Part model, mm, in its own coordinate system. Face numbers are marked on the shaded views. A direction names the side the tool comes from. Round coordinates to 2 decimals unless told otherwise and drop trailing zeros. Write each loop counter-clockwise with the first axis right and the second up, starting at its lowest first coordinate (ties: lowest second). Pieces come first, ordered by that corner, then holes.
from build123d import *

# Parameters (mm, degrees)
SKETCH1_R           = 6.25
BOSS_EXTRUDE1_DEPTH = 3.75
BOSS_EXTRUDE2_DEPTH = 2.5


with BuildPart() as part:
    # Sketch1 → Boss-Extrude1 (new body, symmetric)
    with BuildSketch(Plane.XY):
        with BuildLine():
            ThreePointArc((14.68337521, -5), (23.5795956, -2.206380053), (19, 5.916079783))
            Line((19, 5.916079783), (1.5, 8.874119675))
            ThreePointArc((1.5, 8.874119675), (-1.711171484, 8.835830021), (-4.704473056, 7.672544119))
            ThreePointArc((-4.704473056, 7.672544119), (-14.388421791, 5.006214545), (-23.453994607, 0.681452586))
            Line((-23.453994607, 0.681452586), (-24.470827362, 2.403675322))
            Line((-24.470827362, 2.403675322), (-34.804163773, -3.697321205))
            Line((-34.804163773, -3.697321205), (-29.72, -12.308434881))
            ThreePointArc((-29.72, -12.308434881), (-19.025686771, -7.501050673), (-7.617535769, -4.793031276))
            ThreePointArc((-7.617535769, -4.793031276), (-1.570247279, -8.861959348), (5.50692712, -7.118549971))
            Line((5.50692712, -7.118549971), (14.68337521, -5))
        make_face()
        Circle(SKETCH1_R, mode=Mode.SUBTRACT)
    extrude(amount=BOSS_EXTRUDE1_DEPTH, both=True)

    # Sketch2 → Boss-Extrude2 (add, symmetric)
    with BuildSketch(Plane.XY):
        with BuildLine():
            Line((-28.63346637, -11.690418156), (-24.131806399, -9.129888895))
            Line((-24.131806399, -9.129888895), (-23.968684666, -9.421327611))
            Line((-23.968684666, -9.421327611), (-21.496617767, -13.767462129))
            ThreePointArc((-21.496617767, -13.767462129), (-22.466751825, -17.296987603), (-25.996277299, -16.326853546))
            Line((-25.996277299, -16.326853546), (-28.63346637, -11.690418156))
        make_face()
    extrude(amount=BOSS_EXTRUDE2_DEPTH, both=True)


solid = part.part
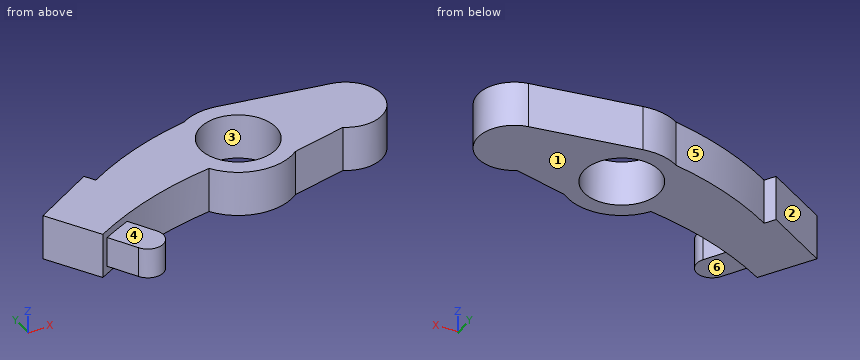
Q1. Saw through at A-A, the plane z = 1. Write the cut outline in (x, y).
Q2. Two-plate mould, pull along X, no slides. Class the marked faces 1, 2 and 3: released by +X, released by -X, zero draft, split by the parting line, or undercut.
Q3. Saw through at D-D, the plane x = 12.5. Write the cut outline in (y, z).
Q4. Saw through at C-C, the plane y = 3.75. Write the cut outline in (x, z), and give its area (3 significant figures).
Q5. Wall check: line 1 (Y direction, x = 0, z = -1.75); line 2 (X direction, y = -3, z = 1.25); line 3 (Y direction, x = -4, z = -0.5). Give the ranges that are in metal, low to high.
Q6. Drop flat-ended pins along their axis: P1, Ø1.5, axis at y = -8, z = 1.5, coming from the -X side; P2, Ø2, axis at x = -15, z = 0.5, coming from the +Y side; P3, Ø6, axis at x = -24, y = -15.5, coming from the +Z side. Give the stop position or say it passes through.
Q7. Tool access for the marked faces 4, 5 and 6: list every direction of +Z, -Z, +X, -X, +Y, -Y with a clear straight run to the whole face (end or side of a thin tool).
Q8. Saw through at B-B, the plane x = 0. Write the cut outline in (y, z).
Computed:
1. outline: (-34.8, -3.7) - (-29.72, -12.31) arc R62 cw to (-28.63, -11.7) - (-26, -16.33) arc R2.59 ccw to (-21.5, -13.77) - (-23.97, -9.42) arc R62 cw to (-7.62, -4.79) arc R9 ccw to (5.51, -7.12) - (14.68, -5) arc R6 ccw (long way) to (19, 5.92) - (1.5, 8.87) arc R9 ccw to (-4.7, 7.67) arc R57 ccw to (-23.45, 0.68) - (-24.47, 2.4) - close; hole circle Ø12.5 at (0, 0)
2. face 1: zero draft
2. face 2: released by -X
2. face 3: undercut
3. outline: (-5.5, -3.75) - (7.01, -3.75) - (7.01, 3.75) - (-5.5, 3.75) - close
4. outline: (-17.48, -3.75) - (-5, -3.75) - (-5, 3.75) - (-17.48, 3.75) - close; (5, -3.75) - (22.68, -3.75) - (22.68, 3.75) - (5, 3.75) - close
4. area: 226 mm2
5. line 1: y = -9 to -6.25, 6.25 to 9
5. line 2: x = -33.62 to -5.48, 5.48 to 23.2
5. line 3: y = -8.06 to -4.8, 4.8 to 8.06
6. P1: stops at x = -32.71
6. P2: stops at y = 5.15
6. P3: stops at z = 2.5
7. face 4: +Z, +X, -Y
7. face 5: +Z, -Z, +Y
7. face 6: -Z, +X, -Y
8. outline: (-9, -3.75) - (-6.25, -3.75) - (-6.25, 3.75) - (-9, 3.75) - close; (6.25, -3.75) - (9, -3.75) - (9, 3.75) - (6.25, 3.75) - close
